from build123d import *

# Parameters (mm, degrees)
SKETCH1_R           = 3
SKETCH1_R_2         = 1.65
BOSS_EXTRUDE1_DEPTH = 670
FILLET1_R           = 2


with BuildPart() as part:
    # Sketch1 → Boss-Extrude1 (new body)
    with BuildSketch(Plane.XY):
        Polygon((-8.46, 9.66), (-4.55, 5.75), (4.55, 5.75), (8.46, 9.66), (8.46, 13.26), (4.35, 13.26), (4.35, 15), (15, 15), (15, 4.35), (13.26, 4.35), (13.26, 8.46), (9.66, 8.46), (5.75, 4.55), (5.75, -4.55), (9.66, -8.46), (13.26, -8.46), (13.26, -4.35), (15, -4.35), (15, -15), (4.35, -15), (4.35, -13.26), (8.46, -13.26), (8.46, -9.59186747), (4.61813253, -5.75), (-4.578313253, -5.75), (-8.420180723, -9.59186747), (-8.420180723, -13.26), (-4.35, -13.26), (-4.35, -15), (-15, -15), (-15, -4.35), (-13.26, -4.35), (-13.26, -8.46), (-9.66, -8.46), (-5.75, -4.55), (-5.75, 4.55), (-9.66, 8.46), (-13.26, 8.46), (-13.26, 4.35), (-15, 4.35), (-15, 15), (-4.35, 15), (-4.35, 13.26), (-8.46, 13.26), align=None)
        Circle(SKETCH1_R, mode=Mode.SUBTRACT)
        with Locations((11.73, 11.73)):
            Circle(SKETCH1_R_2, mode=Mode.SUBTRACT)
        with Locations((11.73, -11.73)):
            Circle(SKETCH1_R_2, mode=Mode.SUBTRACT)
        with Locations((-11.73, -11.73)):
            Circle(SKETCH1_R_2, mode=Mode.SUBTRACT)
        with Locations((-11.73, 11.73)):
            Circle(SKETCH1_R_2, mode=Mode.SUBTRACT)
    extrude(amount=BOSS_EXTRUDE1_DEPTH)

    # Fillet1
    fillet1_edges = [part.edges().sort_by_distance(p)[0] for p in [
        (15, 15, 335),
        (15, -15, 335),
        (-15, -15, 335),
        (-15, 15, 335),
    ]]
    fillet(fillet1_edges, radius=FILLET1_R)


solid = part.part
Can you work these out from the model? Positions are in its coordinate system, mm. Round coordinates to 2 decimals unless told otherwise and drop trailing zeros. Write each question's results on one line, items separated by ' | '. Start each with the question number.
Item 1: If we section it at A-A, the plane z = 71.5: State how many separate pieces and enclosed holes the cut face has, then the cut area to 3 significant figures.
Item 2: Please list where these lines run through material, in increasing order: L1, parallel to X at y = -12, z = 297; L2, parallel to Y at x = -11.73, z = 486.5; L3, parallel to Y at x = -0.25, z = 228.
Item 3: Will these pins go through, and if not, where does the flat tip stop? pin 1 (0.9 mm diameter, centred on x = -14, z = 190.5, fed in from +Y); pin 2 (6 mm diameter, centred on x = -1, z = 160, fed in from -Y); pin 3 (1.5 mm diameter, centred on y = -2.5, z = 411.5, fed in from +X).
Results:
1) separate pieces: 1 | enclosed holes: 5 | area: 326 mm2
2) L1: x = -15 to -13.36, -10.1 to -8.42, 8.46 to 10.1, 13.36 to 15 | L2: y = -15 to -13.38, -10.08 to -8.46, 8.46 to 10.08, 13.38 to 15 | L3: y = -5.75 to -2.99, 2.99 to 5.75
3) pin 1: stops at y = 14.92 | pin 2: stops at y = -5.75 | pin 3: stops at x = 5.75
